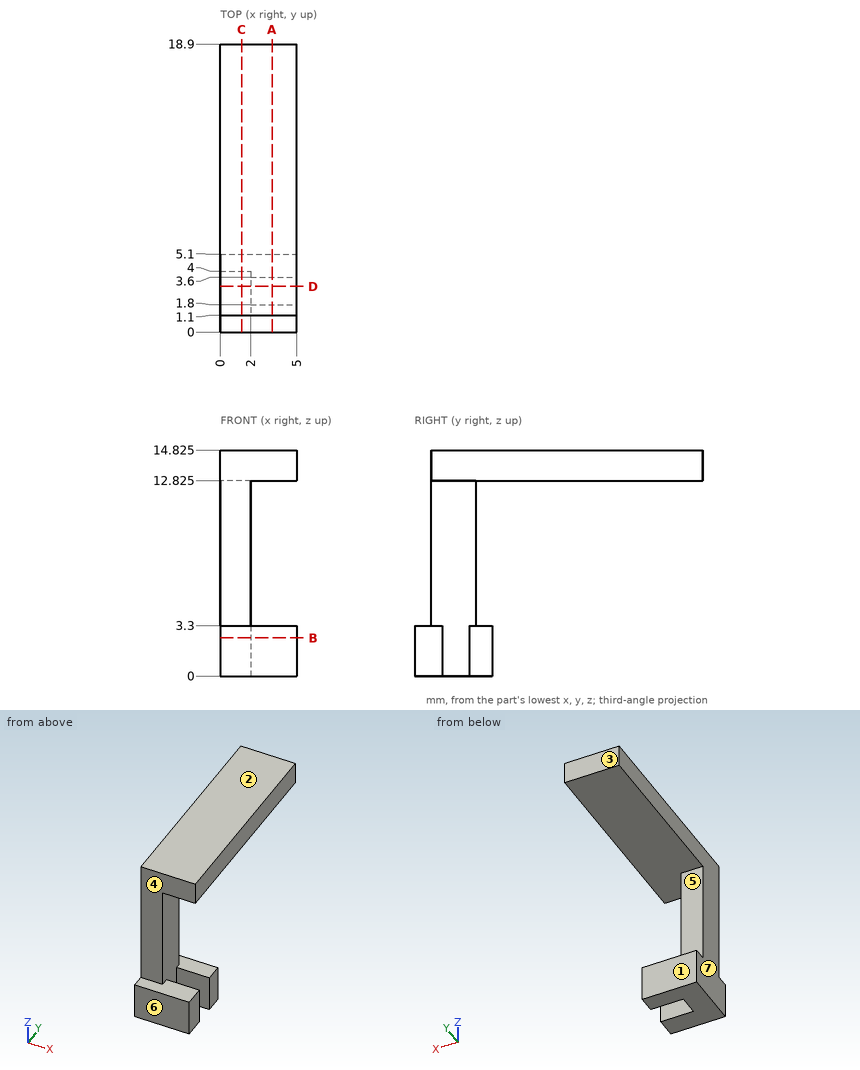
Could you check a few things on this drawing? It's one solid part, dimensions in mm from its lowest x, y, z. A direction names the side the tool comes from. Coordinates: 2 decimals unless noted, no trailing zeros. Order: outer loops, then holes, each group sorted by start corner. A loop starts at its lowest first (then second) coordinate and runs counter-clockwise, first axis right, second up. Notation, with made-up numbers: (5.5, -10) - (39.5, -10) arc R25 cw to (39.5, 25) - close; hole circle Ø4 at (5, 56.5). An arc over 180 degrees is marked (long way). Answer as a JSON object with one key per item and string values. Group by question number.
Q1. Imagine slicing it at C-C (x = 1.4). Please give me the cut outline in (y, z) (3 decimals).
Q2. Imagine slicing it at B-B (z = 2.5). Please give me the cut outline in (x, y), and give its area (3 significant figures).
Q3. Imagine slicing it at A-A (x = 3.4). Please give me the cut outline in (y, z) (3 decimals), and give its area (3 significant figures).
Q4. I need wall thicknesses on line 1 (Y direction, x = 3.7, z = 1.75); line 2 (Z direction, x = 3.3, y = 9.5) (3 decimals); line 3 (Y direction, x = 1.9, z = 2). Which ranges of each line are inside material? Lowest first, please. Write a range as from..to.
Q5. Will these pins go through, and if not, where does the flat tip stop? P1, Ø0.9, axis at x = 3, z = 1.5, coming from the -Y side; P2, Ø0.6, axis at x = 1, z = 8.5, coming from the +Y side; P3, Ø1, axis at x = 3.5, z = 2, coming from the +Y side; P4, Ø0.9, axis at y = 2, z = 8, coming from the +X side.
Q6. On a 3-axis mill with a long thin cutter (end or side, diameter ignored), from which of +Z, -Z, +X, -X, +Y, -Y can I reach the whole of each face in a straight line? I mean the marked faces 1, 2, 3, 4 and 5. Say none if no direction works.
Q7. Imagine slicing it at D-D (y = 3). Please give me the cut outline in (x, z) (3 decimals), and give its area (4 significant figures).
Q8. We'd pull the mould along X, two halves only. Please class the marked faces 6 and 7: +X half, -X half, draft (parallel to the pull), parting line (faces both ways), or undercut.
Determined:
{
 "1": {"outline": "(0, 0) - (5.1, 0) - (5.1, 3.3) - (4, 3.3) - (4, 12.825) - (18.9, 12.825) - (18.9, 14.825) - (1.1, 14.825) - (1.1, 3.3) - (0, 3.3) - close"},
 "2": {"outline": "(0, 0) - (5, 0) - (5, 1.8) - (2, 1.8) - (2, 3.6) - (5, 3.6) - (5, 5.1) - (0, 5.1) - close", "area": "20.1 mm2"},
 "3": {"outline": "(0, 0) - (1.8, 0) - (1.8, 3.3) - (0, 3.3) - close; (1.1, 12.825) - (18.9, 12.825) - (18.9, 14.825) - (1.1, 14.825) - close; (3.6, 0) - (5.1, 0) - (5.1, 3.3) - (3.6, 3.3) - close", "area": "46.5 mm2"},
 "4": {"line 1": "y = 0..1.8, 3.6..5.1", "line 2": "z = 12.825..14.825", "line 3": "y = 0..5.1"},
 "5": {"P1": "stops at y = 0", "P2": "stops at y = 4", "P3": "stops at y = 5.1", "P4": "stops at x = 2"},
 "6": {"face 1": "-Z, +X, -X, +Y", "face 2": "+Z, +X, -X, +Y, -Y", "face 3": "+Z, -Z, +X, -X, +Y", "face 4": "+Z, +X, -X, -Y", "face 5": "+X, -X, +Y"},
 "7": {"outline": "(0, 0) - (2, 0) - (2, 12.825) - (5, 12.825) - (5, 14.825) - (0, 14.825) - close", "area": "35.65 mm2"},
 "8": {"face 6": "draft", "face 7": "-X half"}
}
